Geometry check sheet. Reference: the model listing, model coordinates, mm. Face numbers are marked on the shaded views. A direction names the side the tool comes from. Round coordinates to 2 decimals unless told otherwise and drop trailing zeros. Loops run counter-clockwise (first coordinate to the right, second up) from the corner with the lowest first, then second, coordinate; pieces in that order, holes last. Notation, with made-up numbers: M -13,35.5 L 29,35.5 A10 cw 29,54.5 Z; hole C 59.5,0.5 d11. An arc over 180 degrees is marked long. Write item = value, one per line.
from build123d import *

# Parameters (mm, degrees)
F0_W     = 49
F0_H     = 1.2
F1_DEPTH = 26.99
F2_DEPTH = 42.5
F4_R     = 4
F5_DEPTH = 25
F6_R     = 1.19
F7_DEPTH = 8
F8_R     = 1.19
F9_DEPTH = 8


with BuildPart() as f1:
    # F0 (on Front) → F1 (new body, symmetric)
    with BuildSketch(Plane.XZ):
        with Locations((44.5, 0.6)):
            Rectangle(F0_W, F0_H)
    extrude(amount=F1_DEPTH, both=True)

    # F0 (on Front) → F2 (join, symmetric)
    with BuildSketch(Plane.XZ):
        Polygon((0, 15), (0, 0), (20, 0), (20, 1.2), (20, 15), align=None)
    extrude(amount=F2_DEPTH, both=True)

    # F4 (on offset) → F5 (cut)
    with BuildSketch(Plane.XY.offset(15)):
        with Locations((10, -32.625)):
            Circle(F4_R)
        with Locations((10, 32.625)):
            Circle(F4_R)
    extrude(amount=-F5_DEPTH, mode=Mode.SUBTRACT)

    # F6 (on face) → F7 (cut)
    with BuildSketch(Plane.XZ.offset(42.5)):
        with Locations((10, 7.5)):
            Circle(F6_R)
    extrude(amount=-F7_DEPTH, mode=Mode.SUBTRACT)

    # F8 (on face) → F9 (cut)
    with BuildSketch(Plane(origin=(0, 42.5, 0), x_dir=(-1, 0, 0), z_dir=(0, 1, 0))):
        with Locations((-10, 7.5)):
            Circle(F8_R)
    extrude(amount=-F9_DEPTH, mode=Mode.SUBTRACT)


solid = f1.part
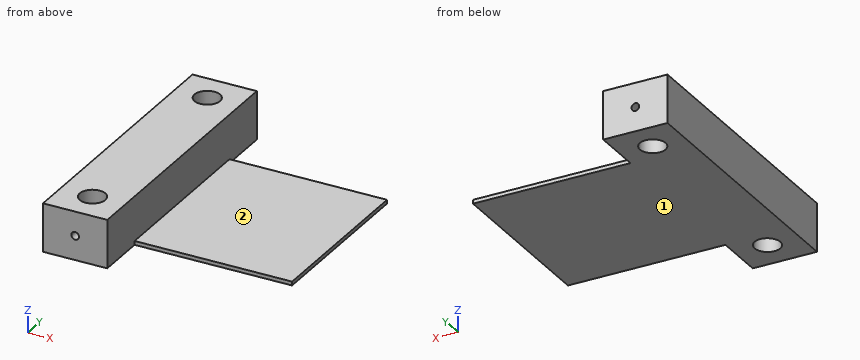
(1) Depth check by flat-ended pin: pin 1 Ø2 at (x, z) = (10, 7.5) entering from -Y; pin 2 Ø1.9 at (x, z) = (10, 7.5) entering from -Y; pin 3 Ø4.5 at (y, z) = (-1.5, 8.5) entering from +X. Enter the tip coordinate at first touch or a pass-through.
Result set:
pin_1 = -28.75
pin_2 = -28.74
pin_3 = 20
(2) Sectioned sample at B-B on z = 7.5. Record the cut outline in (x, y) (3 decimals), then the cut area to 3 significant figures.
Result set:
outline = M 0,-42.5 L 8.81,-42.5 L 8.81,-36.444 A4 cw long 11.19,-36.444 L 11.19,-42.5 L 20,-42.5 L 20,42.5 L 11.19,42.5 L 11.19,36.444 A4 cw long 8.81,36.444 L 8.81,42.5 L 0,42.5 Z
area = 1,570 mm2
(3) Sectioned sample at A-A on x = 10. Record the cut outline in (y, z) (3 decimals).
Result set:
outline = M -42.5,0 L -36.625,0 L -36.625,6.31 L -42.5,6.31 Z; M -42.5,8.69 L -36.625,8.69 L -36.625,15 L -42.5,15 Z; M -28.625,0 L 28.625,0 L 28.625,15 L -28.625,15 Z; M 36.625,0 L 42.5,0 L 42.5,6.31 L 36.625,6.31 Z; M 36.625,8.69 L 42.5,8.69 L 42.5,15 L 36.625,15 Z
(4) Material ranges on line 1 along Y through (x, z) = (12.5, 5.25); line 2 along Y through (x, z) = (13, 13.25); line 3 along Z through (x, y) = (10, -39.75), recorded low to high. Write a range as from..to.
Result set:
line_1 = -42.5..-35.75, -29.5..29.5, 35.75..42.5
line_2 = -42.5..-35.27, -29.98..29.98, 35.27..42.5
line_3 = 0..6.31, 8.69..15
(5) Sectioned sample at C-C on y = 30. Record the cut outline in (x, z).
Result set:
outline = M 0,0 L 6.98,0 L 6.98,15 L 0,15 Z; M 13.02,0 L 20,0 L 20,15 L 13.02,15 Z
(6) Sectioned sample at D-D on y = -16.5. Record the cut outline in (x, z).
Result set:
outline = M 0,0 L 69,0 L 69,1.2 L 20,1.2 L 20,15 L 0,15 Z
(7) Tool access check on the marked faces 1 and 2. Record the directions out of +Z, -Z, +X, -X, +Y, -Y that give a thin tool (end or side, any length) a straight path to the whole face; none if there is none.
Result set:
face_1 = -Z, +X, -X, +Y, -Y
face_2 = +Z, +X, +Y, -Y
